Here's how the part is built. I have some questions about the finished solid (model axes, mm). Face numbers are marked on the shaded views. A direction names the side the tool comes from. Coordinates: 2 decimals unless noted, no trailing zeros. Write each loop counter-clockwise with the first axis right and the second up, starting at its lowest first coordinate (ties: lowest second). Pieces come first, ordered by that corner, then holes.
Item 1: I'm going to push flat-ended pins straight in: P1, Ø7.5, axis at x = 17.5, z = -26, coming from the +Y side; P2, Ø2, axis at x = -1, y = 73.5, coming from the -Z side; P3, Ø8, axis at x = -8.5, y = 70, coming from the +Z side. Where does each tip first touch, or does it pass through?
Item 2: Please list where these lines run through material, in increasing order: line 1 (Y direction, x = -35, z = -70); line 2 (X direction, y = 2, z = -45.5); line 3 (Z direction, x = -28.5, y = 3).
Item 3: If we mould it in two halves opening along Y, with no side actions, what happens to the marked faces 4, 5 and 6? For each: pulls with the +Y half, pulls with the -Y half, needs draft (parallel to the pull), parting line crosses it, or undercut.
Item 4: I want a section at B-B (y = -8.5). Please give me the cut outline in (x, z).
Item 5: For the marked faces 1, 2 and 3, which set-ups out of +Z, -Z, +X, -X, +Y, -Y let a thin tool reach every point of the face, with its end or its side?
Item 6: I want a section at C-C (x = -33.5). Please give me the cut outline in (y, z), and give its area (3 significant figures).
Item 7: I want a section at D-D (z = -39). Please give me the cut outline in (x, y), and give its area (3 significant figures).
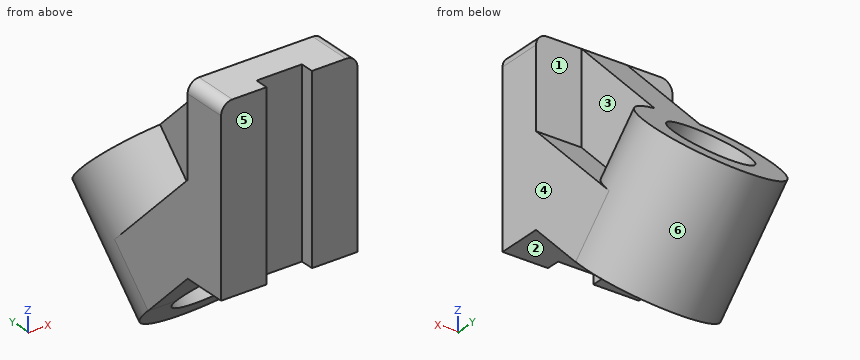
from build123d import *

# Parameters (mm, degrees)
SKETCH1_W                = 76.2
SKETCH1_H                = 25.4
BOSS_EXTRUDE1_DEPTH      = 101.6
BOSS_EXTRUDE2_DEPTH      = 76.2
BOSS_EXTRUDE3_DEPTH      = 35.941
BOSS_EXTRUDE3_DEPTH_BACK = 35.814
SKETCH5_R                = 22.225
CUT_EXTRUDE1_DEPTH       = 148.955
CUT_EXTRUDE2_DEPTH       = 51.724322261
CUT_EXTRUDE3_DEPTH       = 159.487395714


with BuildPart() as part:
    # Sketch1 → Boss-Extrude1 (new body)
    with BuildSketch(Plane.XY):
        with Locations((-8.908273381, -11.00971223)):
            Rectangle(SKETCH1_W, SKETCH1_H)
    extrude(amount=-BOSS_EXTRUDE1_DEPTH)

    # Sketch3 → Boss-Extrude2 (add, through all)
    with BuildSketch(Plane(origin=(29.191726619, 0, 0), x_dir=(0, 0, -1), z_dir=(1, 0, 0))):
        Polygon((50.8, 1.69028777), (106.22230509, 57.112592859), (131.62230509, 31.712592859), (101.6, 1.69028777), align=None)
    extrude(amount=-BOSS_EXTRUDE2_DEPTH)

    # Sketch4 → Boss-Extrude3 (add, two sides)
    with BuildSketch(Plane(origin=(0, -24.554856115, -24.554856115), x_dir=(1, 0, 0), z_dir=(0, 0.707106781, 0.707106781))) as boss_extrude3_sk:
        with BuildLine():
            Line((-21.608273381, 1.195213944), (3.791726619, 1.195213944))
            Line((3.791726619, 1.195213944), (3.791726619, 79.57418946))
            ThreePointArc((3.791726619, 79.57418946), (-8.908273381, 153.595213944), (-21.608273381, 79.57418946))
            Line((-21.608273381, 79.57418946), (-21.608273381, 1.195213944))
        make_face()
    extrude(amount=BOSS_EXTRUDE3_DEPTH)
    extrude(boss_extrude3_sk.sketch, amount=-BOSS_EXTRUDE3_DEPTH_BACK)

    # Sketch5 → Cut-Extrude1 (cut, through all)
    with BuildSketch(Plane(origin=(0, 0.859268708, 0.859268708), x_dir=(1, 0, 0), z_dir=(0, 0.707106781, 0.707106781))):
        with Locations((-8.908273381, 115.495213944)):
            Circle(SKETCH5_R)
    extrude(amount=-CUT_EXTRUDE1_DEPTH, mode=Mode.SUBTRACT)

    # Sketch6 → Cut-Extrude2 (cut, through all)
    with BuildSketch(Plane(origin=(0, 1.69028777, 0), x_dir=(1, 0, 0), z_dir=(0, 1, 0))):
        with BuildLine():
            Line((-47.008273381, 6.35), (-47.008273381, 0))
            Line((-47.008273381, 0), (-40.658273381, 0))
            ThreePointArc((-40.658273381, 0), (-45.148401442, 1.859871939), (-47.008273381, 6.35))
        make_face()
        with BuildLine():
            Line((22.841726619, 0), (29.191726619, 0))
            Line((29.191726619, 0), (29.191726619, 6.35))
            ThreePointArc((29.191726619, 6.35), (27.331854679, 1.859871939), (22.841726619, 0))
        make_face()
    extrude(amount=-CUT_EXTRUDE2_DEPTH, mode=Mode.SUBTRACT)

    # Sketch7 → Cut-Extrude3 (cut, through all)
    with BuildSketch(Plane.XY):
        Polygon((-21.608273381, -23.70971223), (-21.608273381, -16.08971223), (3.791726619, -16.08971223), (3.791726619, -23.70971223), (3.791726619, -49.034034492), (-21.608273381, -49.034034492), align=None)
    extrude(amount=-CUT_EXTRUDE3_DEPTH, mode=Mode.SUBTRACT)


solid = part.part
Answer:
1. P1: stops at y = 1.69
1. P2: stops at z = -143.59
1. P3: stops at z = -64.28
2. line 1: y = -23.71 to 20.89, 54.07 to 71.72
2. line 2: x = -21.61 to 3.79
2. line 3: z = -102.91 to -52.11
3. face 4: needs draft
3. face 5: pulls with the -Y half
3. face 6: undercut
4. outline: (-47.01, -101.6) - (29.19, -101.6) - (29.19, -6.35) arc R6.35 ccw to (22.84, 0) - (-40.66, 0) arc R6.35 ccw to (-47.01, -6.35) - close
5. face 1: +Z, +X, +Y
5. face 2: -Z, +X, -X, -Y
5. face 3: +Z, +X
6. outline: (-23.71, -101.6) - (1.69, -101.6) - (31.71, -131.62) - (31.79, -131.55) - (52.37, -152.12) - (103.1, -101.39) - (61.95, -60.23) - (36.54, -85.64) - (1.69, -50.8) - (1.69, 0) - (-23.71, 0) - close
6. area: 7,880 mm2
7. outline: (-47.01, -23.71) - (-21.61, -23.71) - (-21.61, -16.09) - (3.79, -16.09) - (3.79, -23.71) - (29.19, -23.71) - (29.19, 1.69) - (3.79, 1.69) - (3.79, 40.72) - (-21.61, 40.72) - (-21.61, 1.69) - (-47.01, 1.69) - close
7. area: 2,730 mm2
